CAD build for the part. Positions are in the model's coordinates, mm. A direction names the side the tool comes from. Coordinates: 2 decimals unless noted, no trailing zeros. Loops run counter-clockwise (first coordinate to the right, second up) from the corner with the lowest first, then second, coordinate; pieces in that order, holes last. Notation, with made-up numbers: (13.25, -34.75) -> (59.25, -34.75) arc R20 cw to (59.25, -1.75) -> close; hole circle Ø7 at (-31.75, -18). An arc over 180 degrees is marked (long way). Write item = value, one per line. Start each with the question number.
(1) Band-saw the part on B-B (x = 1). Count the separate pieces of the cut face and the enclosed holes in it, and give its area (3 significant figures).
(2) Band-saw the part on D-D (z = 0). Write the cut outline in (x, y).
(3) Drill centre lines: line 1 (Z direction, x = -0.5, y = 0); line 2 (Y direction, x = 0, z = -2.65); line 3 (Y direction, x = 0, z = 3.5). Where is each one in solid material? Low to high. Write a range as from..to.
(4) Tool access for faces 1 (the face through (-1.957, 11.807, -6.077)), 2 (the face through (0, 13.106, 4)), 3 (the face through (0, 7, 1.003)): list every direction of +Z, -Z, +X, -X, +Y, -Y with a clear straight run to the whole face (end or side of a thin tool).
(5) Band-saw the part on A-A (z = -4.25). Write the cut outline in (x, y), and give its area (3 significant figures).
(6) Pull direction Z, two halves, no side cores. Call faces 4 (the face through (0.07, -4.76, 0.2)), 5 (the face through (-4.762, -6, 0)), 6 (the face through (0, 11, -1.003)), 7 (the face through (0, -3, 7.112)): +Z half, -Z half, draft (parallel to the pull), parting line (faces both ways), or undercut.
(7) Flat gauge pins, fed straight in: P1, Ø4, axis at y = -15.875, z = -3.937, coming from the -X side; P2, Ø4, axis at x = 0, y = 8.74, coming from the -Z side. Where does each tip first touch, or does it go through?
(8) Band-saw the part on C-C (y = 0). Write the cut outline in (x, z), and give its area (3 significant figures).
```python
from build123d import *

# Parameters (mm, degrees)
SKETCH1_W                                          = 31.75
SKETCH1_H                                          = 32.1564
BOSS_EXTRUDE1_DEPTH                                = 9.525
SKETCH2_W                                          = 8.763
SKETCH2_H                                          = 32.1564
CUT_EXTRUDE1_DEPTH                                 = 27.563955842
CUT_EXTRUDE2_DEPTH                                 = 27.563955842
SKETCH4_W                                          = 8.763
SKETCH4_H                                          = 32.16
CUT_EXTRUDE3_DEPTH                                 = 27.563955842
SKETCH5_W                                          = 9.525
SKETCH5_H                                          = 4.7625
SKETCH6_W                                          = 1.3208
SKETCH6_H                                          = 6.1087
CBORE_FOR_M2_5_HEX_HEAD_MACHINE_SCREW1_D           = 3.1
CBORE_FOR_M2_5_HEX_HEAD_MACHINE_SCREW1_CBORE_D     = 7.28
CBORE_FOR_M2_5_HEX_HEAD_MACHINE_SCREW1_CBORE_DEPTH = 2.1
M4X0_7_TAPPED_HOLE1_D                              = 3.3


with BuildPart() as part:
    # Sketch1 → Boss-Extrude1 (new body)
    with BuildSketch(Plane(origin=(4.7625, 0, 0), x_dir=(0, 0, -1), z_dir=(1, 0, 0))):
        with Locations((0, -2.9718)):
            Rectangle(SKETCH1_W, SKETCH1_H)
    extrude(amount=-BOSS_EXTRUDE1_DEPTH)

    # Sketch2 → Cut-Extrude1 (cut, through all)
    with BuildSketch(Plane.ZY.offset(4.7625)):
        with Locations((-11.4935, -2.9718)):
            Rectangle(SKETCH2_W, SKETCH2_H)
    extrude(amount=-CUT_EXTRUDE1_DEPTH, mode=Mode.SUBTRACT)

    # Sketch3 → Cut-Extrude2 (cut, through all)
    with BuildSketch(Plane.ZY.offset(4.7625)):
        with BuildLine():
            Line((1.0033, 13.1064), (-1.0033, 13.1064))
            Line((-1.0033, 13.1064), (-1.0033, 4.655619761))
            ThreePointArc((-1.0033, 4.655619761), (0, 4.7625), (1.0033, 4.655619761))
            Line((1.0033, 4.655619761), (1.0033, 13.1064))
        make_face()
    extrude(amount=-CUT_EXTRUDE2_DEPTH, mode=Mode.SUBTRACT)

    # Sketch4 → Cut-Extrude3 (cut, through all)
    with BuildSketch(Plane.ZY.offset(4.7625)):
        with Locations((11.4935, -2.9736)):
            Rectangle(SKETCH4_W, SKETCH4_H)
    extrude(amount=-CUT_EXTRUDE3_DEPTH, mode=Mode.SUBTRACT)

    # Sketch5 → Cut-Revolve1 (revolve, cut)
    with BuildSketch(Plane.XY):
        with Locations((0, 2.38125)):
            Rectangle(SKETCH5_W, SKETCH5_H)
    revolve(axis=Axis((-4.7625, 0, 0), (1, 0, 0)), mode=Mode.SUBTRACT)

    # Sketch6 → Hole1 (revolve, cut)
    with BuildSketch(Plane(origin=(0, 8.7376, 1.0033), x_dir=(0, 1, 0), z_dir=(1, 0, 0))):
        with Locations((0.6604, 3.05435)):
            Rectangle(SKETCH6_W, SKETCH6_H)
    revolve(axis=Axis((0, 8.7376, 111.0033), (0, 0, -1)), mode=Mode.SUBTRACT)

    # CBORE for M2.5 Hex Head Machine Screw1 (through all)
    with Locations(Plane(origin=(0, 0, -7.112), x_dir=(-1, 0, 0), z_dir=(0, 0, -1))):
        with Locations((0, 8.7376)):
            CounterBoreHole(CBORE_FOR_M2_5_HEX_HEAD_MACHINE_SCREW1_D / 2, CBORE_FOR_M2_5_HEX_HEAD_MACHINE_SCREW1_CBORE_D / 2, CBORE_FOR_M2_5_HEX_HEAD_MACHINE_SCREW1_CBORE_DEPTH)

    # M4x0.7 Tapped Hole1 (through all)
    with Locations(Plane(origin=(4.7625, -17.4625, 0), x_dir=(0, 1, 0), z_dir=(1, 0, 0))):
        with Locations((1.5875, -3.937), (1.5875, 3.937)):
            Hole(M4X0_7_TAPPED_HOLE1_D / 2)


solid = part.part
```
Findings below:
q1.separate_pieces = 3
q1.enclosed_holes = 2
q1.area = 314 mm²
q2.outline = (-4.76, -19.05) -> (4.76, -19.05) -> (4.76, -4.76) -> (-4.76, -4.76) -> close
q3.line_1 = -7.11..-4.76, 4.76..7.11
q3.line_2 = -19.05..-16.91, -14.84..-3.96, 3.96..7.19, 10.29..13.11
q3.line_3 = -19.05..-17.47, -14.28..-3.23, 3.23..7.19, 10.29..13.11
q4.face_1 = -Z
q4.face_2 = +Z, -Z, +X, -X, +Y
q4.face_3 = +X, -X, +Y
q5.outline = (-4.76, -19.05) -> (4.76, -19.05) -> (4.76, -17.5) -> (-4.76, -17.5) -> close; (-4.76, -14.25) -> (4.76, -14.25) -> (4.76, -2.15) -> (-4.76, -2.15) -> close; (-4.76, 2.15) -> (4.76, 2.15) -> (4.76, 13.11) -> (-4.76, 13.11) -> close; hole circle Ø3.1 at (0, 8.74)
q5.area = 227 mm²
q6.face_4 = undercut
q6.face_5 = draft
q6.face_6 = undercut
q6.face_7 = +Z half
q7.P1 = -4.76
q7.P2 = -5.01
q8.outline = (-4.76, -7.11) -> (4.76, -7.11) -> (4.76, -4.76) -> (-4.76, -4.76) -> close; (-4.76, 4.76) -> (4.76, 4.76) -> (4.76, 7.11) -> (-4.76, 7.11) -> close
q8.area = 44.8 mm²
